```python
from build123d import *

# Parameters (mm, degrees)
F0_W     = 431.8
F0_H     = 1092.2
F1_DEPTH = 355.6
F2_W     = 425.45
F2_H     = 1038.225
F3_DEPTH = 352.425
F4_W     = 425.45
F4_H     = 50.8
F5_DEPTH = 352.425
F6_W     = 419.1
F6_H     = 346.075
F7_DEPTH = 47.625
F8_W     = 425.45
F8_H     = 349.25
F9_DEPTH = 47.625


with BuildPart() as f1:
    # F0 (on Front) → F1 (new body)
    with BuildSketch(Plane.XZ):
        Rectangle(F0_W, F0_H)
    extrude(amount=F1_DEPTH)

    # F2 (on face) → F3 (cut)
    with BuildSketch(Plane.XZ.offset(355.6)):
        with Locations((0, -23.8125)):
            Rectangle(F2_W, F2_H)
    extrude(amount=-F3_DEPTH, mode=Mode.SUBTRACT)

    # F4 (on face) → F5 (join, through all)
    with BuildSketch(Plane.XZ.offset(3.175)):
        with Locations((0, 168.275)):
            Rectangle(F4_W, F4_H)
    extrude(amount=F5_DEPTH)

    # F6 (on face) → F7 (cut)
    with BuildSketch(Plane.XY.offset(193.675)):
        with Locations((0, -179.3875)):
            Rectangle(F6_W, F6_H)
    extrude(amount=-F7_DEPTH, mode=Mode.SUBTRACT)

    # F8 (on face) → F9 (cut)
    with BuildSketch(Plane.XY.offset(546.1)):
        with Locations((0, -177.8)):
            Rectangle(F8_W, F8_H)
    extrude(amount=-F9_DEPTH, mode=Mode.SUBTRACT)


solid = f1.part
```
Geometry: final body of the model. Coordinates: model frame, mm. A direction names the side the tool comes from. Give positions to 0.01 mm unless a question says otherwise; leave off trailing zeros. Write each loop counter-clockwise with the first axis right and the second up, starting at its lowest first coordinate (ties: lowest second). Pieces come first, ordered by that corner, then holes.
1. Draft query along Y for faces 5 (the flat face through (212.725, -180, 523)), 6 (the flat face through (-3, 0, 8)), 7 (the flat face through (-3, -182, 495.3)). Return one class per face: released by +Y, released by -Y, zero draft, split by the parting line, or undercut.
2. Reachability of faces 1 (the flat face through (-3, -177, 142.875)), 2 (the flat face through (-212.725, -180, 523)), 3 (the flat face through (-3, -352.425, 170)), 4 (the flat face through (-3, -175, -546.1)) from +Z, -Z, +X, -X, +Y, -Y: full face, straight path, thin tool, end or side. Return the list, or none.
3. Section query B-B, the plane z = -329.5. Return loops of the section in (x, y) (3 decimals).
4. Line query: probe 1 along Z at (x, y) = (176, -126.5) (3 decimals); probe 2 along X at (y, z) = (-326, -26.5) (3 decimals); probe 3 along Y at (x, z) = (149, 20) (3 decimals). Output: solid intervals per line, ascending.
5. Section query A-A, the plane y = -160.5. Return loops of the section in (x, z) (3 decimals), then the cut area to 3 significant figures.
6. Pin query (flat end, axial travel): P1, Ø3, axis at x = -74, z = 204.5, coming from the -Y side (3 decimals); P2, Ø3, axis at x = -168, y = -222.5, coming from the +Z side (3 decimals); P3, Ø1.5, axis at x = -143.5, z = 75, coming from the +Y side. Return the tip coordinate at first contact, or that it passes through.
7. Section query C-C, the plane x = 60. Return loops of the section in (y, z) (3 decimals).
Computed:
1. face 5: undercut
1. face 6: released by +Y
1. face 7: zero draft
2. face 1: -Y
2. face 2: +Z
2. face 3: none
2. face 4: -Z, +X, -X, +Y, -Y
3. outline: (-215.9, -355.6) - (-212.725, -355.6) - (-212.725, -3.175) - (212.725, -3.175) - (212.725, -355.6) - (215.9, -355.6) - (215.9, 0) - (-215.9, 0) - close
4. probe 1: z = -546.1 to -542.925, 142.875 to 146.05, 495.3 to 498.475
4. probe 2: x = -215.9 to -212.725, 212.725 to 215.9
4. probe 3: y = -3.175 to 0
5. outline: (-215.9, -546.1) - (215.9, -546.1) - (215.9, 546.1) - (212.725, 546.1) - (212.725, 498.475) - (-212.725, 498.475) - (-212.725, 546.1) - (-215.9, 546.1) - close; hole (-212.725, -542.925) - (212.725, -542.925) - (212.725, 142.875) - (-212.725, 142.875) - close; hole (-212.725, 193.675) - (-209.55, 193.675) - (-209.55, 146.05) - (209.55, 146.05) - (209.55, 193.675) - (212.725, 193.675) - (212.725, 495.3) - (-212.725, 495.3) - close
5. area: 11,300 mm2
6. P1: stops at y = -3.175
6. P2: stops at z = 498.475
6. P3: stops at y = 0
7. outline: (-355.6, -546.1) - (0, -546.1) - (0, 546.1) - (-3.175, 546.1) - (-3.175, 498.475) - (-352.425, 498.475) - (-352.425, 546.1) - (-355.6, 546.1) - (-355.6, 495.3) - (-3.175, 495.3) - (-3.175, 193.675) - (-6.35, 193.675) - (-6.35, 146.05) - (-352.425, 146.05) - (-352.425, 193.675) - (-355.6, 193.675) - (-355.6, 142.875) - (-3.175, 142.875) - (-3.175, -542.925) - (-355.6, -542.925) - close
